```python
from build123d import *

# Parameters (mm, degrees)
SKETCH1_R           = 15
BOSS_EXTRUDE1_DEPTH = 100
SKETCH3_W           = 15
SKETCH3_H           = 15
CUT_EXTRUDE2_DEPTH  = 75
SKETCH2_R           = 6
BOSS_EXTRUDE2_DEPTH = 40
SKETCH4_R           = 11
BOSS_EXTRUDE3_DEPTH = 5


with BuildPart() as part:
    # Sketch1 → Boss-Extrude1 (new body)
    with BuildSketch(Plane(origin=(0, 0, 0), x_dir=(1, 0, 0), z_dir=(0, 1, 0))):
        Circle(SKETCH1_R)
    extrude(amount=BOSS_EXTRUDE1_DEPTH)

    # Sketch3 → Cut-Extrude2 (cut)
    with BuildSketch(Plane(origin=(0, 100, 0), x_dir=(1, 0, 0), z_dir=(0, 1, 0))):
        Rectangle(SKETCH3_W, SKETCH3_H)
        with BuildLine():
            Line((-7.5, 12.990381057), (-7.5, 7.5))
            Line((-7.5, 7.5), (7.5, 7.5))
            Line((7.5, 7.5), (7.5, 12.990381057))
            ThreePointArc((7.5, 12.990381057), (3.882285677, 14.488887394), (0, 15))
            ThreePointArc((0, 15), (-3.882285677, 14.488887394), (-7.5, 12.990381057))
        make_face()
    extrude(amount=-CUT_EXTRUDE2_DEPTH, mode=Mode.SUBTRACT)

    # Sketch2 → Boss-Extrude2 (add)
    with BuildSketch(Plane.XZ):
        Circle(SKETCH2_R)
    extrude(amount=BOSS_EXTRUDE2_DEPTH)

    # Sketch4 → Boss-Extrude3 (add)
    with BuildSketch(Plane(origin=(0, -40, 0), x_dir=(-1, 0, 0), z_dir=(0, -1, 0))):
        Circle(SKETCH4_R)
    extrude(amount=BOSS_EXTRUDE3_DEPTH)


solid = part.part
```
Read the model definition and answer for the solid it produces. Units are mm, in the model's axes. A direction names the side the tool comes from. Coordinates: 2 decimals unless noted, no trailing zeros. Loops run counter-clockwise (first coordinate to the right, second up) from the corner with the lowest first, then second, coordinate; pieces in that order, holes last.
(1) The mould has two halves that part along X. Classify faces 1 (the face through (0, 100, 10)), 2 (the face through (0, 63, 7.5)), 3 (the face through (-3.252, 49.3, 14.643)): released by +X, released by -X, zero draft, split by the parting line, or undercut.
Solution:
face 1: zero draft
face 2: undercut
face 3: split by the parting line
(2) Flat-ended cylindrical pins translate along their axes: pin 1 Ø3 at (x, y) = (-3, 28) entering from +Z; pin 2 Ø6 at (x, z) = (12, -6) entering from -Y; pin 3 Ø6 at (y, z) = (44, -7.5) entering from -X; pin 4 Ø5 at (x, y) = (-11, 33.5) entering from +Z. Find the tip coordinate at first contact, or state that the pin passes through.
Solution:
pin 1: stops at z = 14.92
pin 2: stops at y = -45
pin 3: stops at x = -14.31
pin 4: stops at z = 12.36
(3) The part is cut by section D-D (y = -24). Determine the outline of the cut face in (x, z).
Solution:
outline: circle Ø12 at (0, 0)
(4) The part is cut by section A-A (z = 0). Determine the outline of the cut face in (x, y), and give its area (4 significant figures).
Solution:
outline: (-15, 0) - (-6, 0) - (-6, -40) - (-11, -40) - (-11, -45) - (11, -45) - (11, -40) - (6, -40) - (6, 0) - (15, 0) - (15, 100) - (7.5, 100) - (7.5, 25) - (-7.5, 25) - (-7.5, 100) - (-15, 100) - close
area: 2,465 mm2
(5) The part is cut by section B-B (x = -2.5). Determine the outline of the cut face in (y, z), and give its area (3 significant figures).
Solution:
outline: (-45, -10.71) - (-40, -10.71) - (-40, -5.45) - (0, -5.45) - (0, -14.79) - (25, -14.79) - (25, 7.5) - (100, 7.5) - (100, 14.79) - (0, 14.79) - (0, 5.45) - (-40, 5.45) - (-40, 10.71) - (-45, 10.71) - close
area: 1,830 mm2
(6) The part is cut by section C-C (y = 58.5). Determine the outline of the cut face in (x, z).
Solution:
outline: (-7.5, -12.99) - (-7.5, 7.5) - (7.5, 7.5) - (7.5, -12.99) arc R15 ccw (long way) to start
(7) A tool of negligible diameter and unlimited length cuts with its end or side. For faces 4 (the face through (2.38, -42.46, 10.74)), 5 (the face through (-6, -20, 0)), 6 (the face through (7.5, 63, -3)), from which of +Z, -Z, +X, -X, +Y, -Y can it reach the whole face along a straight path? Write none if from no direction.
Solution:
face 4: -Y
face 5: none
face 6: -Z, +Y
(8) Consider line 1 along X through (y, z) = (61.5, 0.25); line 2 along Y through (x, z) = (4.25, 9.5); line 3 along Y through (x, z) = (-5, -3.75). Determine where each line is inside the solid, lowest interval first.
Solution:
line 1: x = -15 to -7.5, 7.5 to 15
line 2: y = -45 to -40, 0 to 100
line 3: y = -45 to -40, 0 to 25
